```python
from build123d import *

# Parameters (mm, degrees)
SKETCH_1_R      = 1.5
EXTRUDE_1_DEPTH = 5
SKETCH_2_W      = 25
SKETCH_2_H      = 34
SKETCH_2_R      = 1.5
SKETCH_2_R_2    = 4
SKETCH_2_H_2    = 5
EXTRUDE_2_DEPTH = 5
SKETCH_3_R      = 1.5
EXTRUDE_3_DEPTH = 5


with BuildPart() as part:
    # 스케치1 → 보스-돌출1 (new body)
    with BuildSketch(Plane(origin=(0, 0, 0), x_dir=(1, 0, 0), z_dir=(0, 1, 0))):
        Polygon((12.5, 30), (-12.5, 30), (-25, 14.387505004), (-25, -30), (25, -30), (25, 14.387505004), align=None)
        with Locations(Location((-13.5, 5, 0), (0, 0, 270))):
            Circle(SKETCH_1_R, mode=Mode.SUBTRACT)
        with Locations(Location((-5.24, 25.4, 0), (0, 0, 270))):
            Circle(SKETCH_1_R, mode=Mode.SUBTRACT)
        with Locations(Location((13.5, 5, 0), (0, 0, 270))):
            Circle(SKETCH_1_R, mode=Mode.SUBTRACT)
        with Locations(Location((5.24, 25.4, 0), (0, 0, 270))):
            Circle(SKETCH_1_R, mode=Mode.SUBTRACT)
    extrude(amount=EXTRUDE_1_DEPTH)

    # 스케치2 → 보스-돌출2 (add)
    # profile 1 of 2: a face of its own
    with BuildSketch(Plane.XY.offset(30)):
        with Locations((0, -17)):
            Rectangle(SKETCH_2_W, SKETCH_2_H)
        with Locations((0, -18.5)):
            Circle(SKETCH_2_R, mode=Mode.SUBTRACT)
        with Locations((-7, -11.5)):
            Circle(SKETCH_2_R, mode=Mode.SUBTRACT)
        with Locations((0, -11.5)):
            Circle(SKETCH_2_R_2, mode=Mode.SUBTRACT)
        with Locations((7, -11.5)):
            Circle(SKETCH_2_R, mode=Mode.SUBTRACT)
        with Locations((0, -4.5)):
            Circle(SKETCH_2_R, mode=Mode.SUBTRACT)
    # profile 2 of 2: a face of its own
    with BuildSketch(Plane.XY.offset(30)):
        with Locations((0, 2.5)):
            Rectangle(SKETCH_2_W, SKETCH_2_H_2)
    extrude(amount=EXTRUDE_2_DEPTH)

    # 스케치3 → 보스-돌출3 (add)
    with BuildSketch(Plane(origin=(0, 5, 0), x_dir=(1, 0, 0), z_dir=(0, 1, 0))):
        Polygon((51.2, 14.95), (51.2, -4.95), (25, -4.95), (25, 14.387505004), (24.549643574, 14.95), align=None)
        with Locations(Location((47.7, -2, 0), (0, 0, 270))):
            Circle(SKETCH_3_R, mode=Mode.SUBTRACT)
        with Locations(Location((47.7, 12, 0), (0, 0, 90))):
            Circle(SKETCH_3_R, mode=Mode.SUBTRACT)
    extrude(amount=-EXTRUDE_3_DEPTH)


solid = part.part
```
Work out the finished part from the listing and answer in its coordinate system (mm). A direction names the side the tool comes from. Coordinates: 2 decimals unless noted, no trailing zeros. Loops run counter-clockwise (first coordinate to the right, second up) from the corner with the lowest first, then second, coordinate; pieces in that order, holes last. Notation, with made-up numbers: (-38.5, 86.5) - (14.5, 86.5) arc R21 ccw to (14.5, 121.5) - close; hole circle Ø8 at (42.25, 18.25). An arc over 180 degrees is marked (long way). Use a Markdown table: item, result.
Item 1: Find section D-D, the plane x = 47.7. Determine the outline of the cut face in (y, z), and give its area (3 significant figures).
Evaluation:
| item | result |
|---|---|
| outline | (0, -14.95) - (5, -14.95) - (5, -13.5) - (0, -13.5) - close; (0, -10.5) - (5, -10.5) - (5, 0.5) - (0, 0.5) - close; (0, 3.5) - (5, 3.5) - (5, 4.95) - (0, 4.95) - close |
| area | 69.5 mm2 |
Item 2: The mould has two halves that part along X. Classify faces 4 (the flat face through (-3, -19, 35)), 5 (the cylindrical face through (5.8, -12.4, 32.5)), 6 (the cylindrical face through (49.187, 2.535, 1.805)), 7 (the flat face through (51.2, 3, -5)): +X half, -X half, draft (parallel to the pull), parting line (faces both ways), or undercut.
Evaluation:
| item | result |
|---|---|
| face 4 | draft |
| face 5 | undercut |
| face 6 | undercut |
| face 7 | +X half |
Item 3: Find section A-A, the plane x = 0. Determine the outline of the cut face in (y, z), and give its area (3 significant figures).
Evaluation:
| item | result |
|---|---|
| outline | (-34, 30) - (-20, 30) - (-20, 35) - (-34, 35) - close; (-17, 30) - (-15.5, 30) - (-15.5, 35) - (-17, 35) - close; (-7.5, 30) - (-6, 30) - (-6, 35) - (-7.5, 35) - close; (-3, 30) - (0, 30) - (0, -30) - (5, -30) - (5, 35) - (-3, 35) - close |
| area | 425 mm2 |
Item 4: For faces 1 (the flat face through (-0.2, -16.8, 30)), 2 (the flat face through (38, 3, -14.95)), 3 (the flat face through (25, 2, 18)), determine the directions among +Z, -Z, +X, -X, +Y, -Y from which every point of the face is accessible in a straight line to the end or side of a thin tool.
Evaluation:
| item | result |
|---|---|
| face 1 | -Z, +X, -X, -Y |
| face 2 | -Z, +X, +Y, -Y |
| face 3 | +Z, +X, +Y, -Y |
Item 5: Find section B-B, the plane y = -11.5. Determine the outline of the cut face in (x, z).
Evaluation:
| item | result |
|---|---|
| outline | (-12.5, 30) - (-8.5, 30) - (-8.5, 35) - (-12.5, 35) - close; (-5.5, 30) - (-4, 30) - (-4, 35) - (-5.5, 35) - close; (4, 30) - (5.5, 30) - (5.5, 35) - (4, 35) - close; (8.5, 30) - (12.5, 30) - (12.5, 35) - (8.5, 35) - close |
Item 6: Given pin 1 Ø2.5 at (x, y) = (19, 3.5) entering from +Z; pin 2 Ø18 at (x, z) = (31.5, -11.5) entering from -Y; pin 3 Ø6 at (y, z) = (-28.5, 27.5) entering from -X; pin 4 Ø2.5 at (x, y) = (7, -11.5) entering from -Z, each flat-ended and moving along its own axis, determine where each tip first touches the part or whether it passes through.
Evaluation:
| item | result |
|---|---|
| pin 1 | stops at z = 30 |
| pin 2 | stops at y = 0 |
| pin 3 | stops at x = -12.5 |
| pin 4 | passes through |
Item 7: Find section C-C, the plane z = -5. Determine the outline of the cut face in (x, y), and give its area (3 significant figures).
Evaluation:
| item | result |
|---|---|
| outline | (-25, 0) - (-15, 0) - (-15, 5) - (-25, 5) - close; (-12, 0) - (12, 0) - (12, 5) - (-12, 5) - close; (15, 0) - (51.2, 0) - (51.2, 5) - (15, 5) - close |
| area | 351 mm2 |
Item 8: Consider probe 1 along Y at (x, z) = (0, 32); probe 2 along X at (y, z) = (2.3, -5); probe 3 along X at (y, z) = (1.5, 2). Determine where each line is inside the solid, lowest interval first. Write a range as from..to.
Evaluation:
| item | result |
|---|---|
| probe 1 | y = -34..-20, -17..-15.5, -7.5..-6, -3..5 |
| probe 2 | x = -25..-15, -12..12, 15..51.2 |
| probe 3 | x = -25..46.2, 49.2..51.2 |
